Check sheet for the drawn part. Datum: minimum x, y, z corner. Units: mm. A direction names the side the tool comes from. Coordinates: 2 decimals unless noted, no trailing zeros. Order: outer loops, then holes, each group sorted by start corner. A loop starts at its lowest first (then second) coordinate and runs counter-clockwise, first axis right, second up.
Q1. Cross-section at A-A, the plane x = 42.5. Record the boundary of the cut face in (y, z).
Q2. Cross-section at D-D, the plane x = 7. Record the boundary of the cut face in (y, z), and give its area (3 significant figures).
Q3. Cross-section at B-B, the plane x = 27.5. Record the boundary of the cut face in (y, z), and give its area (3 significant figures).
Q4. Thickness scan on line 1 (X direction, y = 8.75, z = 7.5); line 2 (Z direction, x = 22.5, y = 16); line 3 (Y direction, x = 7, z = 6). Record the ranges inside material, lowest first.
Q5. Cross-section at C-C, the plane z = 24. Record the boundary of the cut face in (x, y), and give its area (3 significant figures).
Q6. Set-up check for the marked faces 1 and 2: record each of +Z, -Z, +X, -X, +Y, -Y from which the full face is reachable in a straight line by a thin tool's end or side.
Q7. Draft check along Z on the marked faces 3, 4, 5 and 6. Enter one of: pulls with the +Z half, pulls with the -Z half, needs draft (parallel to the pull), parting line crosses it, or undercut.
Q8. Depth check by flat-ended pin: P1, Ø2, axis at y = 11.5, z = 11, coming from the +X side; P2, Ø2, axis at y = 3, z = 25, coming from the +X side. Enter the tip coordinate at first touch or a pass-through.
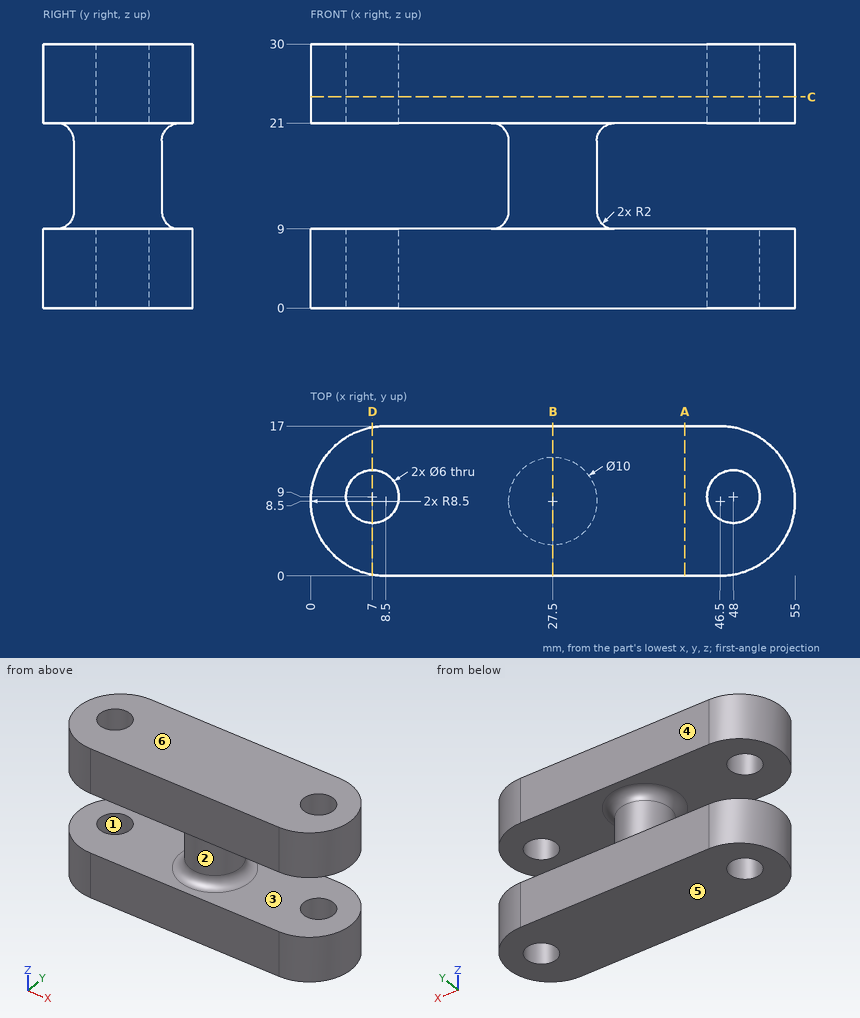
Check values:
1. outline: (0, 0) - (17, 0) - (17, 9) - (0, 9) - close; (0, 21) - (17, 21) - (17, 30) - (0, 30) - close
2. outline: (0.13, 0) - (6, 0) - (6, 9) - (0.13, 9) - close; (0.13, 21) - (6, 21) - (6, 30) - (0.13, 30) - close; (12, 0) - (16.87, 0) - (16.87, 9) - (12, 9) - close; (12, 21) - (16.87, 21) - (16.87, 30) - (12, 30) - close
2. area: 193 mm2
3. outline: (0, 0) - (17, 0) - (17, 9) - (15.5, 9) arc R2 cw to (13.5, 11) - (13.5, 19) arc R2 cw to (15.5, 21) - (17, 21) - (17, 30) - (0, 30) - (0, 21) - (1.5, 21) arc R2 cw to (3.5, 19) - (3.5, 11) arc R2 cw to (1.5, 9) - (0, 9) - close
3. area: 429 mm2
4. line 1: x = 0 to 4.01, 9.99 to 45.01, 50.99 to 55
4. line 2: z = 0 to 9, 21 to 30
4. line 3: y = 0.13 to 6, 12 to 16.87
5. outline: (8.5, 0) - (46.5, 0) arc R8.5 ccw to (46.5, 17) - (8.5, 17) arc R8.5 ccw to start; hole circle Ø6 at (7, 9); hole circle Ø6 at (48, 9)
5. area: 816 mm2
6. face 1: +Z, -Z
6. face 2: none
7. face 3: undercut
7. face 4: needs draft
7. face 5: pulls with the -Z half
7. face 6: pulls with the +Z half
8. P1: stops at x = 32.09
8. P2: stops at x = 53.71
